from build123d import *

# Parameters (mm, degrees)
BOSS_EXTRUDE1_DEPTH = 6.35
CUT_EXTRUDE1_REACH  = 37.786
SKETCH2_R           = 2.032
CUT_EXTRUDE2_REACH  = 37.786
SKETCH3_R           = 2.032
FILLET2_R           = 1.27
LPATTERN1_COUNT     = 2
LPATTERN1_PITCH     = 7.62


with BuildPart() as part:
    # Sketch1 → Boss-Extrude1 (new, symmetric)
    with BuildSketch(Plane.XY):
        Polygon((0, 0), (0, 16.256), (10.16, 16.256), (10.16, 3.175), (31.242, 3.175), (31.242, 0), align=None)
    extrude(amount=BOSS_EXTRUDE1_DEPTH, both=True)

    # Sketch2 → Cut-Extrude1 (cut, up to next)
    with BuildSketch(Plane.ZY, mode=Mode.PRIVATE) as cut_extrude1_sk1:
        with Locations((0, 8.89)):
            Circle(SKETCH2_R)
    cut_extrude1_tool1 = extrude(cut_extrude1_sk1.sketch, amount=-CUT_EXTRUDE1_REACH, mode=Mode.PRIVATE) & part.part
    add(cut_extrude1_tool1.solids().sort_by_distance((0, 8.89, 0))[0], mode=Mode.SUBTRACT)

    # Sketch3 → Cut-Extrude2 (cut, up to next)
    with BuildSketch(Plane.XZ, mode=Mode.PRIVATE) as cut_extrude2_sk1:
        with Locations((18.542, 0)):
            Circle(SKETCH3_R)
    cut_extrude2_tool1 = extrude(cut_extrude2_sk1.sketch, amount=-CUT_EXTRUDE2_REACH, mode=Mode.PRIVATE) & part.part
    cut_extrude2 = cut_extrude2_tool1.solids().sort_by_distance((18.542, 0, 0))[0]
    add(cut_extrude2, mode=Mode.SUBTRACT)

    # Fillet2
    fillet2_edges = [part.edges().sort_by_distance(p)[0] for p in [
        (10.16, 3.175, 0),
    ]]
    fillet(fillet2_edges, radius=FILLET2_R)

    # LPattern1: Cut-Extrude2 ×2
    with Locations(*[(i * LPATTERN1_PITCH, 0, 0) for i in range(1, LPATTERN1_COUNT)]):
        add(cut_extrude2, mode=Mode.SUBTRACT)


solid = part.part
Check sheet for the modelled part. Datum: model origin and axes. Units: mm. A direction names the side the tool comes from. Round coordinates to 2 decimals unless told otherwise and drop trailing zeros. Write each loop counter-clockwise with the first axis right and the second up, starting at its lowest first coordinate (ties: lowest second). Pieces come first, ordered by that corner, then holes. Notation, with made-up numbers: (-27, 46) -> (3, 46) arc R34 ccw to (3, 80) -> close; hole circle Ø11 at (-35, 67). An arc over 180 degrees is marked (long way). Answer as CSV lines item,"result". Start each with the question number.
1) Material ranges on line 1 (X direction, y = 11, z = 4.75); line 2 (Y direction, x = 21, z = 1.25) (3 decimals); line 3 (Y direction, x = 2.75, z = 0), recorded low to high. Write a range as from..to.
2) Section check A-A on z = 0. Enter the section's corners in (x, y) (3 decimals), and give its area (3 significant figures).
3) Section check D-D on y = 6. Enter the section's corners in (x, z).
4) Release check for a two-part mould opening along X. For faces 3 (the flat face through (9, 6, -6.35)), 4 (the flat face through (31.242, 2, 0)), 5 (the cylindrical face through (20.48, 1.57, 0.61)) record: pulls with the +X half, pulls with the -X half, needs draft (parallel to the pull), parting line crosses it, or undercut.
5) Section check B-B on y = 8.89. Enter the section's corners in (x, z), and give its area (3 significant figures).
6) Section check C-C on z = 3.75. Enter the section's corners in (x, y) (3 decimals).
7) Tool access check on faces 1 (the flat face through (10.16, 12, 0)), 2 (the flat face through (5, 16.256, 0)). Record the directions out of +Z, -Z, +X, -X, +Y, -Y that give a thin tool (end or side, any length) a straight path to the whole face; none if there is none.
8) Go/stop test with flat-tipped pins: P1, Ø2, axis at x = 11.5, z = 4, coming from the +Y side; P2, Ø3.5, axis at x = 18.542, z = 0, coming from the +Y side; P3, Ø6.5, axis at x = 22, z = 3, coming from the +Y side (3 decimals). Record where each tip stops, or that it passes through.
Found:
1,line 1,"x = 0..10.16"
1,line 2,"y = 0..3.175"
1,line 3,"y = 0..6.86, 10.92..16.26"
2,outline,"(0, 0) -> (16.51, 0) -> (16.51, 3.175) -> (11.43, 3.175) arc R1.27 cw to (10.16, 4.445) -> (10.16, 6.858) -> (0, 6.858) -> close; (0, 10.922) -> (10.16, 10.922) -> (10.16, 16.256) -> (0, 16.256) -> close; (20.574, 0) -> (24.13, 0) -> (24.13, 3.175) -> (20.574, 3.175) -> close; (28.194, 0) -> (31.242, 0) -> (31.242, 3.175) -> (28.194, 3.175) -> close"
2,area,"165 mm^2"
3,outline,"(0, -6.35) -> (10.16, -6.35) -> (10.16, 6.35) -> (0, 6.35) -> close"
4,face 3,"needs draft"
4,face 4,"pulls with the +X half"
4,face 5,"undercut"
5,outline,"(0, -6.35) -> (10.16, -6.35) -> (10.16, -2.03) -> (0, -2.03) -> close; (0, 2.03) -> (10.16, 2.03) -> (10.16, 6.35) -> (0, 6.35) -> close"
5,area,"87.7 mm^2"
6,outline,"(0, 0) -> (31.242, 0) -> (31.242, 3.175) -> (11.43, 3.175) arc R1.27 cw to (10.16, 4.445) -> (10.16, 16.256) -> (0, 16.256) -> close"
7,face 1,"+Z, -Z, +X, +Y"
7,face 2,"+Z, -Z, +X, -X, +Y"
8,P1,"stops at y = 3.58"
8,P2,"passes through"
8,P3,"stops at y = 3.175"
